```python
from build123d import *

# Parameters (mm, degrees)
PROFILE_DEPTH      = 6.35
CUT_EXTRUDE1_DEPTH = 99.192500569


with BuildPart() as part:
    # Sketch1 → Profile (new body)
    with BuildSketch(Plane.XY):
        Polygon((-44.7548, 79.375), (-44.7548, 73.025), (-51.1048, 73.025), (-51.1048, 69.841302271), (-54.2798, 69.841302271), (-54.2798, 73.025), (-57.4548, 73.025), (-57.4548, 66.675), (-44.7548, 66.675), (-44.7548, 47.625), (-57.4548, 47.625), (-57.4548, 41.275), (-54.2798, 41.275), (-54.2798, 44.458697729), (-51.1048, 44.458697729), (-51.1048, 41.275), (-44.7548, 41.275), (-44.7548, 34.925), (0, -22.225), (0, -15.875), (6.35, -15.875), (6.35, -12.691302271), (9.525, -12.691302271), (9.525, -15.875), (12.7, -15.875), (12.7, -9.525), (0, -9.525), (0, 9.525), (12.7, 9.525), (12.7, 15.875), (9.525, 15.875), (9.525, 12.691302271), (6.35, 12.691302271), (6.35, 15.875), (0, 15.875), (0, 22.225), align=None)
    extrude(amount=PROFILE_DEPTH)

    # Sketch2 → Cut-Extrude1 (cut, through all)
    with BuildSketch(Plane.XY.offset(6.35)):
        Polygon((-31.623026277, 45.530869772), (-36.622463702, 41.615754776), (-28.792233709, 31.616879926), (-23.792796284, 35.531994923), align=None)
        Polygon((-15.962566291, 25.533120074), (-8.132336298, 15.534245224), (-13.131773723, 11.619130228), (-20.962003716, 21.618005077), align=None)
    extrude(amount=-CUT_EXTRUDE1_DEPTH, mode=Mode.SUBTRACT)


solid = part.part
```
Part model, mm, in its own coordinate system. A direction names the side the tool comes from. Give positions to 0.01 mm unless a question says otherwise; leave off trailing zeros. Order: outer loops, then holes, each group sorted by start corner. A loop starts at its lowest first (then second) coordinate and runs counter-clockwise, first axis right, second up. Notation, with made-up numbers: M -8.75,-26 L 40.25,-26 A29 cw 40.25,-1 Z; hole C 25.25,5 d2. An arc over 180 degrees is marked long. Use a Markdown table: item, result. Add a question column.
(1) 3-axis set-ups, long thin cutter, end or side, ignore diameter. For faces 5 (the face through (-44.755, 76, 3)), 6 (the face through (-51, 66.675, 3)), 7 (the face through (9.525, -14, 3)): which of +Z, -Z, +X, -X, +Y, -Y reach the whole face in a straight line?
(2) Mould opens along X. For faces 1 (the face through (-20, 25, 0)), 2 (the face through (-27.65, 40.46, 3.22)), 3 (the face through (-22.064, 50.4, 3.131)), 4 (the face through (-22.69, 6.75, 3.13)) say: +X half, -X half, draft (parallel to the pull), parting line (faces both ways), or undercut.
(3) Drop flat-ended pins along their axis: P1, Ø3.5, axis at x = -52.5, z = 2.5, coming from the -Y side (3 decimals); P2, Ø1.9, axis at x = -49, z = 4, coming from the +Y side (3 decimals); P3, Ø1, axis at x = 10.5, z = 1.5, coming from the -Y side (3 decimals). Give the stop position or say it passes through.
(4) Saw through at C-C, the plane z = 3. Give the number of separate pieces and of enclosed holes in the cut face, and give its area (3 significant figures).
(5) Probe line 1 along Y through (x, z) = (1, 5) (3 decimals); line 2 along Y through (x, z) = (-51, 3.25) (3 decimals); line 3 along X through (y, z) = (41.5, 1.5). List the from-to ranges inside material, lowest first. Write a range as [from, to].
(6) Saw through at B-B, the plane x = -33.5. Give the cut face in (y, z).
(7) Saw through at D-D, the plane y = 14.5. Give the cut face in (x, z) (3 decimals).
(8) Saw through at A-A, the plane y = 40. Give the cut face in (x, z).
Answer key:
| question | item | result |
|---|---|---|
| 1 | face 5 | +Z, -Z, -X, +Y |
| 1 | face 6 | +Z, -Z, -X |
| 1 | face 7 | +Z, -Z, -Y |
| 2 | face 1 | draft |
| 2 | face 2 | undercut |
| 2 | face 3 | +X half |
| 2 | face 4 | -X half |
| 3 | P1 | y = 41.275 |
| 3 | P2 | y = 73.025 |
| 3 | P3 | y = -15.875 |
| 4 | separate pieces | 1 |
| 4 | enclosed holes | 2 |
| 4 | area | 2,110 mm^2 |
| 5 | line 1 | [-15.875, -9.525], [9.525, 15.875] |
| 5 | line 2 | [41.275, 47.625], [66.675, 73.025] |
| 5 | line 3 | [-57.45, -54.28], [-51.1, -36.53], [-28.47, -15.09] |
| 6 | outline | M 20.55,0 L 37.63,0 L 37.63,6.35 L 20.55,6.35 Z; M 44.06,0 L 65,0 L 65,6.35 L 44.06,6.35 Z |
| 7 | outline | M -28.76,0 L -15.388,0 L -15.388,6.35 L -28.76,6.35 Z; M -9.453,0 L 6.35,0 L 6.35,6.35 L -9.453,6.35 Z; M 9.525,0 L 12.7,0 L 12.7,6.35 L 9.525,6.35 Z |
| 8 | outline | M -44.75,0 L -35.36,0 L -35.36,6.35 L -44.75,6.35 Z; M -27.29,0 L -13.92,0 L -13.92,6.35 L -27.29,6.35 Z |
